Autodesk Inventor part; units mm, degrees
ref_plane "YZ Plane" through (0, 0, 0) normal (1, 0, 0) x (0, 1, 0)
ref_plane "XZ Plane" through (0, 0, 0) normal (0, 1, 0) x (-1, 0, 0)
ref_plane "XY Plane" through (0, 0, 0) normal (0, 0, 1) x (1, 0, 0)
sketch "Sketch1" plane through (0, 0, 0) normal (0, 0, 1) x (1, 0, 0)
  line L0 (0, 0) -> (12, 0)
  line L1 (12, 0) -> (12, 10)
  line L2 (12, 10) -> (0, 10)
  line L3 (0, 10) -> (0, 0)
  dimension "d0" = 12
  dimension "d1" = 10
extrude "Extrusion1" add sketch "Sketch1" along normal blind 600
sketch "Sketch3" plane through (0, 0, 600) normal (0, 0, 1) x (1, 0, 0)
  line L0 (12, 10) -> (0, 10)
  line L1 (1, 1) -> (11, 1)
  line L2 (11, 1) -> (11, 9)
  line L3 (11, 9) -> (1, 9)
  line L4 (1, 9) -> (1, 1)
  line L5 (11, 1) -> (1, 9) construction
  point P0 (0, 0)
  point P1 (6, 5)
extrude "Extrusion3" cut sketch "Sketch3" against normal through all
sketch "Sketch5" plane through (0, 0, 0) normal (0, -1, 0) x (1, 0, 0)
  circle A0 centre (6, 10) radius 3
  point P0 (0, 0)
  dimension "d12" = 6
extrude "Extrusion4" cut sketch "Sketch5" against normal through all
properties part number "perfil aluminio"
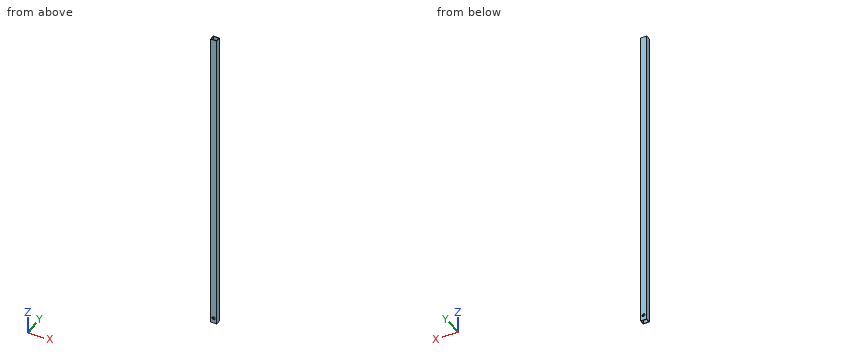
Input: part model. Units: mm. Frame: model coordinates. Round coordinates to 2 decimals unless told otherwise and drop trailing zeros. Write each loop counter-clockwise with the first axis right and the second up, starting at its lowest first coordinate (ties: lowest second). Pieces come first, ordered by that corner, then holes.
1) Cut plane B-B (y = 5.5). Return the cut outline in (x, z).
2) Contact query for a flat-ended pin moving along its axis: P1, Ø5.5, axis at x = 6, z = 10, coming from the +Y side. Output: stop coordinate, or through.
3) Ray query, L1, parallel to Y at x = 7.25, z = 502; L2, parallel to Z at x = 6, y = 0.2; L3, parallel to X at y = 4.5, z = 206.5. Return the intervals inside material, ascending.
4) Cut plane A-A (x = 6). Return the cut outline in (y, z), then the cut area to 3 significant figures.
5) Cut plane C-C (z = 479). Return the cut outline in (x, y).
Geometry says:
1. outline: (0, 0) - (1, 0) - (1, 600) - (0, 600) - close; (11, 0) - (12, 0) - (12, 600) - (11, 600) - close
2. P1: passes through
3. L1: y = 0 to 1, 9 to 10
3. L2: z = 0 to 7, 13 to 600
3. L3: x = 0 to 1, 11 to 12
4. outline: (0, 0) - (1, 0) - (1, 7) - (0, 7) - close; (0, 13) - (1, 13) - (1, 600) - (0, 600) - close; (9, 0) - (10, 0) - (10, 7) - (9, 7) - close; (9, 13) - (10, 13) - (10, 600) - (9, 600) - close
4. area: 1,190 mm2
5. outline: (0, 0) - (12, 0) - (12, 10) - (0, 10) - close; hole (1, 1) - (11, 1) - (11, 9) - (1, 9) - close
